```python
from build123d import *

# Parameters (mm, degrees)
CROQUIS1_W              = 38.1
CROQUIS1_H              = 38.1
SALIENTE_EXTRUIR1_DEPTH = 150
CROQUIS4_W              = 35.7
CROQUIS4_H              = 35.7
CORTAR_EXTRUIR3_DEPTH   = 300
CROQUIS2_R              = 6.25
CORTAR_EXTRUIR5_DEPTH   = 10


with BuildPart() as part:
    # Croquis1 → Saliente-Extruir1 (new body)
    with BuildSketch(Plane.XY):
        Rectangle(CROQUIS1_W, CROQUIS1_H)
    extrude(amount=SALIENTE_EXTRUIR1_DEPTH)

    # Croquis4 → Cortar-Extruir3 (cut)
    with BuildSketch(Plane(origin=(0, 0, 0), x_dir=(-1, 0, 0), z_dir=(0, 0, -1))):
        Rectangle(CROQUIS4_W, CROQUIS4_H)
    extrude(amount=-CORTAR_EXTRUIR3_DEPTH, mode=Mode.SUBTRACT)

    # Croquis2 → Cortar-Extruir5 (cut)
    with BuildSketch(Plane(origin=(19.05, 0, 0), x_dir=(0, 0, -1), z_dir=(1, 0, 0))):
        with Locations(Location((-40, 0, 0), (0, 0, 90))):
            Circle(CROQUIS2_R)
        with BuildLine():
            Line((-128, -6.25), (-84, -6.25))
            ThreePointArc((-84, -6.25), (-77.75, 0), (-84, 6.25))
            Line((-84, 6.25), (-128, 6.25))
            ThreePointArc((-128, 6.25), (-134.25, 0), (-128, -6.25))
        make_face()
    extrude(amount=-CORTAR_EXTRUIR5_DEPTH, mode=Mode.SUBTRACT)


solid = part.part
```
The listing builds one solid part. Answer for the finished solid, in the listing's coordinates (mm). A direction names the side the tool comes from. Give positions to 0.01 mm unless a question says otherwise; leave off trailing zeros. Order: outer loops, then holes, each group sorted by start corner. A loop starts at its lowest first (then second) coordinate and runs counter-clockwise, first axis right, second up. Notation, with made-up numbers: M -4.75,9 L 0.25,9 A19 ccw 0.25,22 Z; hole C 25,-33.5 d5. An arc over 180 degrees is marked long. Put each result on its own line as item: value. Start each with the question number.
Item 1: The part is cut by section D-D, the plane z = 95.5. Determine the outline of the cut face in (x, y).
Item 2: The part is cut by section B-B, the plane x = 2.5. Determine the outline of the cut face in (y, z).
Item 3: The part is cut by section A-A, the plane y = 0. Determine the outline of the cut face in (x, z).
Item 4: Which of the six approach directions +Z, -Z, +X, -X, +Y, -Y give full straight-line access (tool end or side, diameter ignored) to faces 1 (the face through (17.85, 0, 74)), 2 (the face through (19.05, 0, 74)), 3 (the face through (18.46, 0.14, 134.25))?
Item 5: For a pull along Z with two mould halves and no side action, classify faces 4 (the face through (18.46, -0.14, 77.75)), 5 (the face through (-1.5, -18.3, 0)), 6 (the face through (0, -17.85, 74)) as +Z half, -Z half, draft (parallel to the pull), parting line (faces both ways), or undercut.
Item 6: Find the intervals of material crossed by line 1 along Z through (x, y) = (18.15, 0); line 2 along Y through (x, z) = (-14, 14), in increasing order.
Item 7: A flat-ended cylindrical pin translates along its axis: P1, Ø10, axis at y = -2, z = 118, coming from the +X side. Find the tip coordinate at first contact, or state that the pin passes through.
Answer key:
1. outline: M -19.05,-19.05 L 19.05,-19.05 L 19.05,-6.25 L 17.85,-6.25 L 17.85,-17.85 L -17.85,-17.85 L -17.85,17.85 L 17.85,17.85 L 17.85,6.25 L 19.05,6.25 L 19.05,19.05 L -19.05,19.05 Z
2. outline: M -19.05,0 L -17.85,0 L -17.85,150 L -19.05,150 Z; M 17.85,0 L 19.05,0 L 19.05,150 L 17.85,150 Z
3. outline: M -19.05,0 L -17.85,0 L -17.85,150 L -19.05,150 Z; M 17.85,0 L 19.05,0 L 19.05,33.75 L 17.85,33.75 Z; M 17.85,46.25 L 19.05,46.25 L 19.05,77.75 L 17.85,77.75 Z; M 17.85,134.25 L 19.05,134.25 L 19.05,150 L 17.85,150 Z
4. face 1: +Z, -Z
4. face 2: +Z, -Z, +X, +Y, -Y
4. face 3: +X
5. face 4: undercut
5. face 5: -Z half
5. face 6: draft
6. line 1: z = 0 to 33.75, 46.25 to 77.75, 134.25 to 150
6. line 2: y = -19.05 to -17.85, 17.85 to 19.05
7. P1: stops at x = 19.05
